Answer from the drawing. Dimensions are ordinates in mm from the lowest x, y and z of the part. Coordinates: 2 decimals unless noted, no trailing zeros. Write each loop counter-clockwise with the first axis right and the second up, starting at its lowest first coordinate (ties: lowest second). Pieces come first, ordered by that corner, then holes.
(1) For a pull along Y with two mould halves and no side action, classify the marked faces 1, 2 and 3 as +Y half, -Y half, draft (parallel to the pull), parting line (faces both ways), or undercut.
(2) Straight lines are drawn through the part: line 1 (Y direction, x = 15, z = 3.5); line 2 (X direction, y = 14.75, z = 6.5); line 3 (X direction, y = 22.75, z = 2.75). For each, find the intervals that lie inside material, in ascending order.
(3) The part is cut by section C-C on z = 5.75. Determine the outline of the cut face in (x, y), plus the area to 3 significant figures.
(4) The part is cut by section A-A on y = 15. Determine the outline of the cut face in (x, z), plus the area to 4 significant figures.
(5) The part is cut by section B-B on x = 15. Determine the outline of the cut face in (y, z).
(6) Given P1, Ø1, axis at y = 6.5, z = 4.5, coming from the -X side; P2, Ø2, axis at x = 15, y = 15, coming from the +Z side; P3, Ø2, axis at x = 25, z = 3, coming from the +Y side; P4, Ø2, axis at x = 15.5, z = 4.5, coming from the -Y side, each flat-ended and moving along its own axis, determine where each tip first touches the part or whether it passes through.
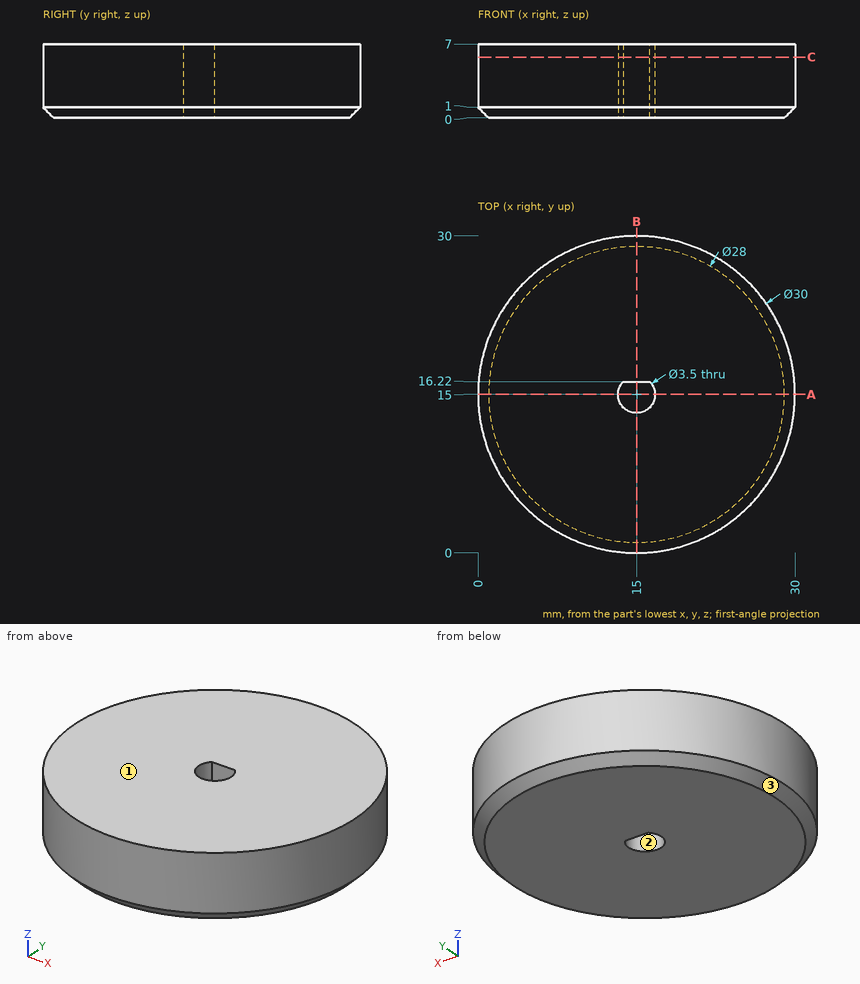
Model answer:
1. face 1: draft
1. face 2: undercut
1. face 3: parting line
2. line 1: y = 0 to 13.25, 16.22 to 30
2. line 2: x = 0 to 13.27, 16.73 to 30
2. line 3: x = 2.16 to 27.84
3. outline: circle Ø30 at (15, 15); hole (13.75, 16.22) arc R1.75 ccw (long way) to (16.25, 16.22) - close
3. area: 698 mm2
4. outline: (0, 1) - (1, 0) - (13.25, 0) - (13.25, 7) - (0, 7) - close; (16.75, 0) - (29, 0) - (30, 1) - (30, 7) - (16.75, 7) - close
4. area: 184.5 mm2
5. outline: (0, 1) - (1, 0) - (13.25, 0) - (13.25, 7) - (0, 7) - close; (16.22, 0) - (29, 0) - (30, 1) - (30, 7) - (16.22, 7) - close
6. P1: stops at x = 2.31
6. P2: passes through
6. P3: stops at y = 27
6. P4: stops at y = 0
